Source: CAD feature listing. Evaluate the final solid. Frame: model axes, mm. A direction names the side the tool comes from. Round coordinates to 2 decimals unless told otherwise and drop trailing zeros. Order: outer loops, then holes, each group sorted by start corner. A loop starts at its lowest first (then second) coordinate and runs counter-clockwise, first axis right, second up. Notation, with made-up numbers: (-19.5, -36) -> (11.5, -36) arc R22 cw to (11.5, -14) -> close; hole circle Ø3 at (-30.5, 40). An arc over 180 degrees is marked (long way). Answer as CSV lines item,"result". Start each with the question number.
(1) Line query: line 1 along Z through (x, y) = (3.75, 25.5); line 2 along Z through (x, y) = (1.15, 27); line 3 along Y through (x, z) = (2.2, -3.5). Output: solid intervals per line, ascending. Write a range as from..to.
(2) Section query C-C (z = 13.5). Output: boundary loops of the cut face in (x, y) (3 decimals), plus the area to 3 significant figures.
(3) Section query B-B (y = 22). Output: boundary loops of the cut face in (x, z) (3 decimals).
(4) Contact query for flat-ended pins moving along their axis: P1, Ø2, axis at x = 3, z = -14.5, coming from the +Y side; P2, Ø1, axis at x = 3.5, z = -12, coming from the +Y side; P3, Ø2, axis at x = 2, z = -20, coming from the +Y side. Output: stop coordinate, or through.
(5) Section query A-A (x = 1.2). Output: boundary loops of the cut face in (y, z), plus the area to 3 significant figures.
(6) Section query D-D (y = 36.5). Output: boundary loops of the cut face in (x, z) (3 decimals).
(7) Set-up query: faces 1 (the flat face through (2.19, 17.93, 4.14)), 2 (the flat face through (2.254, 25.281, 24.345)), 3 (the cylindrical face through (2.254, 0.362, -30.098)). Return all of +Z, -Z, +X, -X, +Y, -Y with unobstructed straight access to the full face (end or side cutting, diameter ignored); none if empty.
```python
from build123d import *

# Parameters (mm, degrees)
BOSS_EXTRUDE1_DEPTH = 4.445
BOSS_EXTRUDE2_DEPTH = 4.445
FILLET1_R           = 0.889
FILLET2_R           = 1.27
CUT_EXTRUDE1_DEPTH  = 50.624972926
FILLET3_R           = 1.27


with BuildPart() as part:
    # Sketch1 → Boss-Extrude1 (new body)
    with BuildSketch(Plane(origin=(0, 0, 0), x_dir=(0, 0, -1), z_dir=(1, 0, 0))):
        Polygon((0, 0), (30.48, 0), (30.48, 6.35), (-1.792103412, 35.267324495), (-8.142103412, 35.267324495), align=None)
    extrude(amount=BOSS_EXTRUDE1_DEPTH)

    # Sketch2 → Boss-Extrude2 (add)
    with BuildSketch(Plane(origin=(4.445, 0, 0), x_dir=(0, 0, -1), z_dir=(1, 0, 0))):
        Polygon((-8.142103412, 35.267324495), (-25.71389316, 31.210557181), (-22.85701477, 18.836057358), (-25.950639726, 18.121837761), (-29.521737714, 33.589962539), (-5.984546816, 39.023951226), (-1.792103412, 35.267324495), align=None)
    extrude(amount=-BOSS_EXTRUDE2_DEPTH)

    # Fillet1
    fillet1_edges = [part.edges().sort_by_distance(p)[0] for p in [
        (2.2225, 31.210557181, 25.71389316),
        (2.2225, 35.267324495, 8.142103412),
    ]]
    fillet(fillet1_edges, radius=FILLET1_R)

    # Fillet2
    fillet2_edges = [part.edges().sort_by_distance(p)[0] for p in [
        (2.2225, 39.023951226, 5.984546816),
        (2.2225, 33.589962539, 29.521737714),
        (2.2225, 18.121837761, 25.950639726),
        (2.2225, 18.836057358, 22.85701477),
        (2.2225, 6.35, -30.48),
        (2.2225, 0, -30.48),
        (2.2225, 0, 0),
    ]]
    fillet(fillet2_edges, radius=FILLET2_R)

    # Sketch3 → Cut-Extrude1 (cut, through all)
    with BuildSketch(Plane(origin=(4.445, 0, 0), x_dir=(0, 0, -1), z_dir=(1, 0, 0))):
        Polygon((-3.37912104, 31.57359901), (3.030610843, 3.81), (27.605409997, 3.81), align=None)
    extrude(amount=-CUT_EXTRUDE1_DEPTH, mode=Mode.SUBTRACT)

    # Fillet3
    fillet3_edges = [part.edges().sort_by_distance(p)[0] for p in [
        (2.2225, 31.57359901, 3.37912104),
        (2.2225, 3.81, -27.605409997),
        (2.2225, 3.81, -3.030610843),
    ]]
    fillet(fillet3_edges, radius=FILLET3_R)


solid = part.part
```
Answer block:
1,line 1,"-9.11..-3.4, 1.98..5.89, 24.4..27.65"
1,line 2,"-7.43..-1.73, 2.32..6.23, 24.74..28"
1,line 3,"0..3.93, 25.41..30.53"
2,outline,"(0, 34.03) -> (4.445, 34.03) -> (4.445, 37.289) -> (0, 37.289) -> close"
2,area,"14.5 mm2"
3,outline,"(0, -13.014) -> (4.445, -13.014) -> (4.445, -7.305) -> (0, -7.305) -> close; (0, 1.169) -> (4.445, 1.169) -> (4.445, 5.079) -> (0, 5.079) -> close; (0, 23.587) -> (4.445, 23.587) -> (4.445, 26.846) -> (0, 26.846) -> close"
4,P1,"y = 21.56"
4,P2,"y = 23.36"
4,P3,"y = 16.64"
5,outline,"(0, -29.21) arc R1.27 ccw to (1.27, -30.48) -> (5.78, -30.48) arc R1.27 ccw to (6.73, -30.06) -> (38.58, 5.49) arc R1.27 ccw to (38.88, 6.63) -> (33.88, 28.28) arc R1.27 ccw to (32.35, 29.24) -> (19.36, 26.24) arc R1.27 ccw to (18.41, 24.71) -> (18.55, 24.09) arc R1.27 ccw to (20.07, 23.14) -> (30.34, 25.51) arc R0.89 cw to (31.41, 24.85) -> (35.07, 9.01) arc R0.89 cw to (34.4, 7.94) -> (0.98, 0.23) arc R1.27 ccw to (0, -1.01) -> close; hole (3.81, -24.28) arc R1.27 ccw to (6.03, -25.13) -> (28.9, 0.39) arc R1.27 ccw to (27.67, 2.48) -> (4.79, -2.8) arc R1.27 ccw to (3.81, -4.04) -> close"
5,area,"539 mm2"
6,outline,"(0, 3.168) -> (4.445, 3.168) -> (4.445, 16.917) -> (0, 16.917) -> close"
7,face 1,"+X, -X, -Y"
7,face 2,"+X, -X"
7,face 3,"-Z, +X, -X, -Y"
